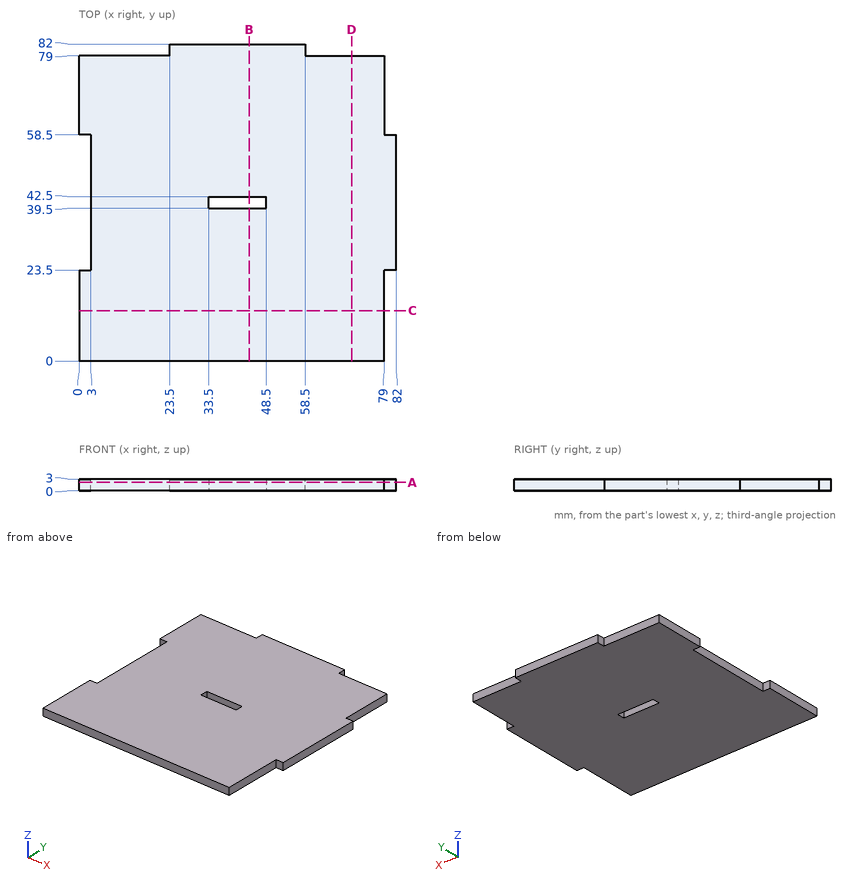
Source: three-view drawing plus pictorial views. Frame: mm from the lowest corner of the part. Coordinates: 2 decimals unless noted, no trailing zeros. Loops run counter-clockwise (first coordinate to the right, second up) from the corner with the lowest first, then second, coordinate; pieces in that order, holes last. Notation, with made-up numbers: (20.5, 54.25) - (72.5, 54.25) arc R16 ccw to (72.5, 61.25) - close; hole circle Ø3 at (-15.5, 63.5). An arc over 180 degrees is marked (long way). Answer in a Markdown table with one row per item. Add a question column.
Item 1: Contact query for flat-ended pins moving along their axis: P1, Ø5, axis at x = 10.5, y = 67.5, coming from the -Z side; P2, Ø1.5, axis at y = 80, z = 2, coming from the -X side; P3, Ø1.5, axis at x = 1.5, z = 1, coming from the +Y side; P4, Ø0.9, axis at x = 80.5, z = 2, coming from the +Y side. Output: stop coordinate, or through.
Item 2: Section query B-B on x = 44. Return the cut outline in (y, z).
Item 3: Section query A-A on z = 2.15. Return the cut outline in (x, y), then the cut area to 3 significant figures.
Item 4: Section query C-C on y = 13. Return the cut outline in (x, z), then the cut area to 3 significant figures.
Item 5: Line query: line 1 along Y through (x, z) = (72, 1.7); line 2 along X through (y, z) = (51, 1.2). Output: solid intervals per line, ascending. Write a range as [from, to].
Recorded:
| question | item | result |
|---|---|---|
| 1 | P1 | z = 0 |
| 1 | P2 | x = 23.5 |
| 1 | P3 | y = 79 |
| 1 | P4 | y = 58.5 |
| 2 | outline | (0, 0) - (39.5, 0) - (39.5, 3) - (0, 3) - close; (42.5, 0) - (82, 0) - (82, 3) - (42.5, 3) - close |
| 3 | outline | (0, 0) - (79, 0) - (79, 23.5) - (82, 23.5) - (82, 58.5) - (79, 58.5) - (79, 79) - (58.5, 79) - (58.5, 82) - (23.5, 82) - (23.5, 79) - (0, 79) - (0, 58.5) - (3, 58.5) - (3, 23.5) - (0, 23.5) - close; hole (33.5, 39.5) - (48.5, 39.5) - (48.5, 42.5) - (33.5, 42.5) - close |
| 3 | area | 6,300 mm^2 |
| 4 | outline | (0, 0) - (79, 0) - (79, 3) - (0, 3) - close |
| 4 | area | 237 mm^2 |
| 5 | line 1 | [0, 79] |
| 5 | line 2 | [3, 82] |
